For this review, use the dimensioned drawing (mm, ordinates from the lowest corner) and the shaded views. Coordinates: 2 decimals unless noted, no trailing zeros. Write each loop counter-clockwise with the first axis right and the second up, starting at its lowest first coordinate (ties: lowest second). Pieces come first, ordered by that corner, then holes. Notation, with made-up numbers: (-36.75, 7) - (5.25, 7) arc R26 cw to (5.25, 36) - close; hole circle Ø7 at (26, 25). An arc over 180 degrees is marked (long way). One line per item, written item: value.
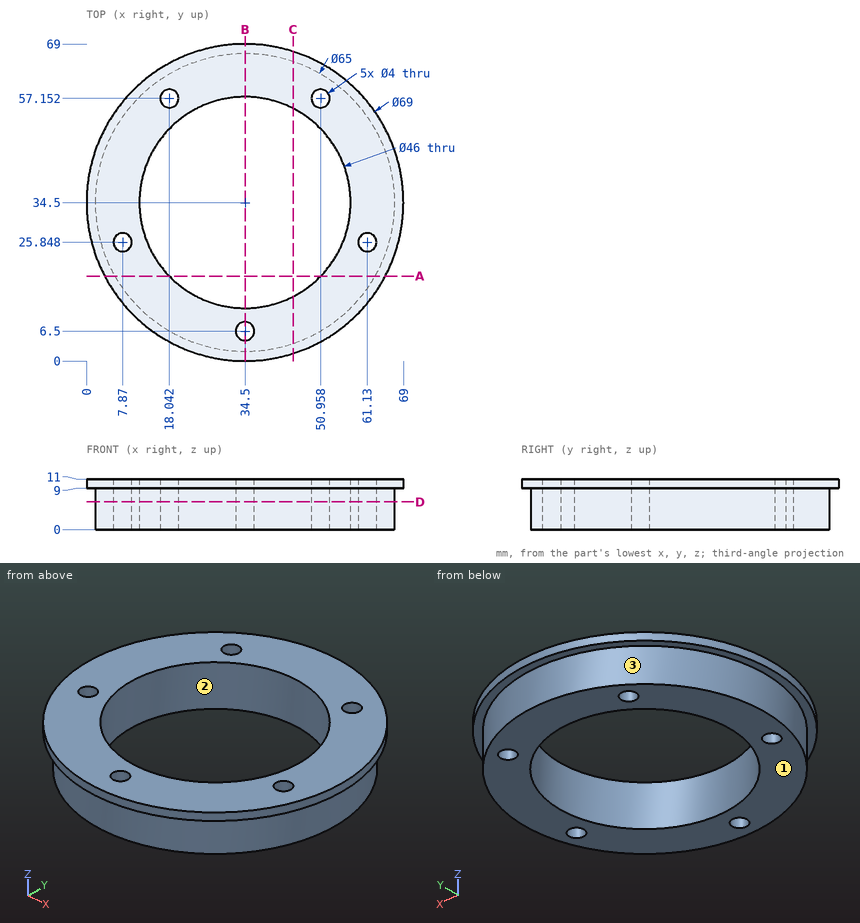
1. Consider section B-B, the plane x = 34.5. Write out the cut boundary in (y, z), then the cut area to 3 significant figures.
Answer block:
outline: (0, 9) - (2, 9) - (2, 0) - (4.5, 0) - (4.5, 11) - (0, 11) - close; (8.5, 0) - (11.5, 0) - (11.5, 11) - (8.5, 11) - close; (57.5, 0) - (67, 0) - (67, 9) - (69, 9) - (69, 11) - (57.5, 11) - close
area: 173 mm^2
2. Consider section C-C, the plane x = 45. Write out the cut boundary in (y, z), then the cut area to 3 significant figures.
Answer block:
outline: (1.64, 9) - (3.74, 9) - (3.74, 0) - (14.04, 0) - (14.04, 11) - (1.64, 11) - close; (54.96, 0) - (65.26, 0) - (65.26, 9) - (67.36, 9) - (67.36, 11) - (54.96, 11) - close
area: 235 mm^2
3. Consider section D-D, the plane z = 6. Write out the cut boundary in (x, y).
Answer block:
outline: circle Ø65 at (34.5, 34.5); hole circle Ø4 at (7.87, 25.85); hole circle Ø46 at (34.5, 34.5); hole circle Ø4 at (18.04, 57.15); hole circle Ø4 at (34.5, 6.5); hole circle Ø4 at (50.96, 57.15); hole circle Ø4 at (61.13, 25.85)
4. Insertion check: pin 1 Ø1.5 at (x, z) = (41.5, 7) entering from -Y; pin 2 Ø2 at (x, z) = (39, 5.5) entering from +Y; pin 3 Ø5 at (y, z) = (53.5, 3.5) entering from -X. Each pin has a flat end and moves straight along its axis. Give the tip position at first contact, or say it passes through.
Answer block:
pin 1: stops at y = 2.61
pin 2: stops at y = 66.81
pin 3: stops at x = 6.5
5. Consider section A-A, the plane y = 18.5. Write out the cut boundary in (x, z) (1 decimal).
Answer block:
outline: (3.9, 9) - (6.2, 9) - (6.2, 0) - (18, 0) - (18, 11) - (3.9, 11) - close; (51, 0) - (62.8, 0) - (62.8, 9) - (65.1, 9) - (65.1, 11) - (51, 11) - close
6. Wall thickness on line 1 along Y through (x, z) = (34.5, 3); line 2 along Y through (x, z) = (19.5, 5) (1 decimal); line 3 along Z through (x, y) = (59, 58): over which ranges is each line inside the solid? List them lowest first.
Answer block:
line 1: y = 2 to 4.5, 8.5 to 11.5, 57.5 to 67
line 2: y = 5.7 to 17.1, 51.9 to 55.8, 58.5 to 63.3
line 3: z = 9 to 11
7. Mouldability with a two-part tool opening along X and no side actions: class the marked faces 1, 2 and 3 as released by +X, released by -X, zero draft, split by the parting line, or undercut.
Answer block:
face 1: zero draft
face 2: undercut
face 3: split by the parting line
